```python
from build123d import *

# Parameters (mm, degrees)
F1_DEPTH = 50


with BuildPart() as f1:
    # F0 (on Top) → F1 (new body)
    with BuildSketch(Plane.XY):
        with BuildLine():
            ThreePointArc((0, 20), (-14.142136, 14.142136), (-20, 0))
            Line((-20, 0), (-20, -20))
            Line((-20, -20), (0, -20))
            Line((0, -20), (20, 0))
            Line((20, 0), (4.226497, 4.226497))
            Line((4.226497, 4.226497), (0, 20))
        make_face()
    extrude(amount=F1_DEPTH)


solid = f1.part
```
Check sheet for the modelled part. Datum: model origin and axes. Units: mm. Round coordinates to 2 decimals unless told otherwise and drop trailing zeros. Order: outer loops, then holes, each group sorted by start corner. A loop starts at its lowest first (then second) coordinate and runs counter-clockwise, first axis right, second up.
1) Go/stop test with flat-tipped pins: pin 1 Ø8 at (y, z) = (13, 18.5) entering from +X; pin 2 Ø2 at (x, z) = (-1.5, 23) entering from +Y. Record where each tip stops, or that it passes through.
2) Section check A-A (z = 5). Record the boundary of the cut face in (x, y), and give its area (3 significant figures).
3) Section check B-B (y = -3). Record the boundary of the cut face in (x, z), and give its area (3 significant figures).
4) Section check C-C (x = 10). Record the boundary of the cut face in (y, z).
5) Scan lines: line 1 (Y direction, x = 6.5, z = 35); line 2 (Y direction, x = -4, z = 9); line 3 (X direction, y = -2, z = 23.5). Record each from-to range of solid material in increasing order.
Result:
1. pin 1: stops at x = 2.95
1. pin 2: stops at y = 19.99
2. outline: (-20, -20) - (0, -20) - (20, 0) - (4.23, 4.23) - (0, 20) arc R20 ccw to (-20, 0) - close
2. area: 999 mm2
3. outline: (-20, 0) - (17, 0) - (17, 50) - (-20, 50) - close
3. area: 1,850 mm2
4. outline: (-10, 0) - (2.68, 0) - (2.68, 50) - (-10, 50) - close
5. line 1: y = -13.5 to 3.62
5. line 2: y = -20 to 19.6
5. line 3: x = -20 to 18
